CAD build for the part. Positions are in the model's coordinates, mm. Coordinates: 2 decimals unless noted, no trailing zeros. Write each loop counter-clockwise with the first axis right and the second up, starting at its lowest first coordinate (ties: lowest second). Pieces come first, ordered by that corner, then holes. Notation, with made-up numbers: M 66.25,10 L 99.25,10 A30 ccw 99.25,47 Z; hole C -21.5,85.25 d1. An arc over 180 degrees is marked long. Put each result on its own line as item: value. Start each with the question number.
```python
from build123d import *

# Parameters (mm, degrees)
SKETCH1_W           = 30
SKETCH1_H           = 10
SKETCH1_R           = 2.3
SKETCH1_R_2         = 2.35
SKETCH1_R_3         = 2.4
SKETCH1_R_4         = 2.45
BOSS_EXTRUDE1_DEPTH = 7
FILLET1_R           = 3


with BuildPart() as part:
    # Sketch1 → Boss-Extrude1 (new body)
    with BuildSketch(Plane(origin=(0, 0, 0), x_dir=(1, 0, 0), z_dir=(0, 1, 0))):
        with Locations((15, 5)):
            Rectangle(SKETCH1_W, SKETCH1_H)
        with Locations(Location((4.5, 5, 0), (0, 0, 270))):
            Circle(SKETCH1_R, mode=Mode.SUBTRACT)
        with Locations(Location((11.5, 5, 0), (0, 0, 270))):
            Circle(SKETCH1_R_2, mode=Mode.SUBTRACT)
        with Locations(Location((18.5, 5, 0), (0, 0, 270))):
            Circle(SKETCH1_R_3, mode=Mode.SUBTRACT)
        with Locations(Location((25.5, 5, 0), (0, 0, 270))):
            Circle(SKETCH1_R_4, mode=Mode.SUBTRACT)
    extrude(amount=BOSS_EXTRUDE1_DEPTH)

    # Fillet1
    fillet1_edges = [part.edges().sort_by_distance(p)[0] for p in [
        (0, 3.5, -10),
        (0, 3.5, 0),
    ]]
    fillet(fillet1_edges, radius=FILLET1_R)


solid = part.part
```
(1) Slice it at B-B, the plane z = -5. Write the cut outline in (x, y), then the cut area to 3 significant figures.
(2) Slice it at C-C, the plane y = 3.25. Write the cut outline in (x, z).
(3) Slice it at A-A, the plane x = 11.5. Write the cut outline in (y, z), then the cut area to 3 significant figures.
(4) Two-plate mould, pull along Z, no slides. Class faces 1 (the face through (15, 7, -5)), 2 (the face through (16, 3, 0)), 3 (the face through (2.255, 3.451, -5.499)): +Z half, -Z half, draft (parallel to the pull), parting line (faces both ways), or undercut.
(5) Drill centre lines: line 1 (X direction, y = 2, z = -5); line 2 (X direction, y = 5.5, z = -5.75); line 3 (Z direction, x = 25, y = 5.5). Where is each one in solid material? Low to high. Write a range as [from, to].
(6) Slice it at D-D, the plane x = 18.5. Write the cut outline in (y, z), then the cut area to 3 significant figures.
Result set:
1. outline: M 0,0 L 2.2,0 L 2.2,7 L 0,7 Z; M 6.8,0 L 9.15,0 L 9.15,7 L 6.8,7 Z; M 13.85,0 L 16.1,0 L 16.1,7 L 13.85,7 Z; M 20.9,0 L 23.05,0 L 23.05,7 L 20.9,7 Z; M 27.95,0 L 30,0 L 30,7 L 27.95,7 Z
1. area: 77.0 mm^2
2. outline: M 0,-7 A3 ccw 3,-10 L 30,-10 L 30,0 L 3,0 A3 ccw 0,-3 Z; hole C 4.5,-5 d4.6; hole C 11.5,-5 d4.7; hole C 18.5,-5 d4.8; hole C 25.5,-5 d4.9
3. outline: M 0,-10 L 7,-10 L 7,-7.35 L 0,-7.35 Z; M 0,-2.65 L 7,-2.65 L 7,0 L 0,0 Z
3. area: 37.1 mm^2
4. face 1: draft
4. face 2: +Z half
4. face 3: undercut
5. line 1: x = [0, 2.2], [6.8, 9.15], [13.85, 16.1], [20.9, 23.05], [27.95, 30]
5. line 2: x = [0, 2.33], [6.67, 9.27], [13.73, 16.22], [20.78, 23.17], [27.83, 30]
5. line 3: z = [-10, -7.4], [-2.6, 0]
6. outline: M 0,-10 L 7,-10 L 7,-7.4 L 0,-7.4 Z; M 0,-2.6 L 7,-2.6 L 7,0 L 0,0 Z
6. area: 36.4 mm^2
